Check sheet for the modelled part. Datum: model origin and axes. Units: mm. A direction names the side the tool comes from. Round coordinates to 2 decimals unless told otherwise and drop trailing zeros. Write each loop counter-clockwise with the first axis right and the second up, starting at its lowest first coordinate (ties: lowest second). Pieces come first, ordered by that corner, then holes. Notation, with made-up numbers: (-11.5, 64) -> (47.5, 64) arc R29 ccw to (47.5, 96) -> close; hole circle Ø4 at (40.5, 77.25). An arc over 180 degrees is marked (long way). Answer as a JSON object with one key per item and string values. Group by question number.
```python
from build123d import *

# Parameters (mm, degrees)
CROQUIS2_W              = 85
CROQUIS2_H              = 85
SALIENTE_EXTRUIR1_DEPTH = 110
CROQUIS3_W              = 20
CROQUIS3_H              = 85
CROQUIS3_W_2            = 7
CORTAR_EXTRUIR1_DEPTH   = 2
CROQUIS5_W              = 83
CROQUIS5_H              = 20
CROQUIS5_H_2            = 7
CORTAR_EXTRUIR2_DEPTH   = 2
CROQUIS6_W              = 20
CROQUIS6_H              = 83
CROQUIS6_W_2            = 7
CORTAR_EXTRUIR3_DEPTH   = 2
CROQUIS7_W              = 81
CROQUIS7_H              = 20
CROQUIS7_H_2            = 7
CORTAR_EXTRUIR4_DEPTH   = 2
CORTAR_EXTRUIR6_DEPTH   = 2
CROQUIS12_W             = 9
CROQUIS12_H             = 9
CORTAR_EXTRUIR7_DEPTH   = 2.5
SALIENTE_EXTRUIR3_DEPTH = 10
SALIENTE_EXTRUIR4_DEPTH = 10
SALIENTE_EXTRUIR5_DEPTH = 10
CROQUIS20_W             = 10
CROQUIS20_H             = 10
SALIENTE_EXTRUIR6_DEPTH = 25
CROQUIS21_W             = 150.699966202
CROQUIS21_H             = 120.747177889
CORTAR_EXTRUIR9_DEPTH   = 112
CROQUIS22_W             = 210
CROQUIS22_H             = 195
SALIENTE_EXTRUIR7_DEPTH = 15
CROQUIS23_W             = 208
CROQUIS23_H             = 195
CROQUIS23_W_2           = 188
CROQUIS23_H_2           = 175
EXTRUIR_L_MINA1_DEPTH   = 110
SALIENTE_EXTRUIR8_REACH = 234.166
CROQUIS25_R             = 15
SALIENTE_EXTRUIR8_DRAFT = -10
CROQUIS26_R             = 5
SALIENTE_EXTRUIR9_DEPTH = 10


with BuildPart() as part:
    # Croquis2 → Saliente-Extruir1 (new body)
    with BuildSketch(Plane.XY):
        Rectangle(CROQUIS2_W, CROQUIS2_H)
    extrude(amount=SALIENTE_EXTRUIR1_DEPTH)

    # Croquis3 → Cortar-Extruir1 (cut)
    with BuildSketch(Plane.ZY.offset(42.5)):
        with Locations((100, 0)):
            Rectangle(CROQUIS3_W, CROQUIS3_H)
        with Locations((81.5, 0)):
            Rectangle(CROQUIS3_W_2, CROQUIS3_H)
        with Locations((69.5, 0)):
            Rectangle(CROQUIS3_W_2, CROQUIS3_H)
    extrude(amount=-CORTAR_EXTRUIR1_DEPTH, mode=Mode.SUBTRACT)

    # Croquis5 → Cortar-Extruir2 (cut)
    with BuildSketch(Plane(origin=(0, 42.5, 0), x_dir=(1, 0, 0), z_dir=(0, 1, 0))):
        with Locations((1, -100)):
            Rectangle(CROQUIS5_W, CROQUIS5_H)
        with Locations((1, -81.5)):
            Rectangle(CROQUIS5_W, CROQUIS5_H_2)
        with Locations((1, -69.5)):
            Rectangle(CROQUIS5_W, CROQUIS5_H_2)
    extrude(amount=-CORTAR_EXTRUIR2_DEPTH, mode=Mode.SUBTRACT)

    # Croquis6 → Cortar-Extruir3 (cut)
    with BuildSketch(Plane(origin=(42.5, 0, 0), x_dir=(0, 0, -1), z_dir=(1, 0, 0))):
        with Locations((-100, -1)):
            Rectangle(CROQUIS6_W, CROQUIS6_H)
        with Locations((-81.5, -1)):
            Rectangle(CROQUIS6_W_2, CROQUIS6_H)
        with Locations((-69.5, -1)):
            Rectangle(CROQUIS6_W_2, CROQUIS6_H)
    extrude(amount=-CORTAR_EXTRUIR3_DEPTH, mode=Mode.SUBTRACT)

    # Croquis7 → Cortar-Extruir4 (cut)
    with BuildSketch(Plane(origin=(0, -42.5, 0), x_dir=(-1, 0, 0), z_dir=(0, -1, 0))):
        with Locations((0, -100)):
            Rectangle(CROQUIS7_W, CROQUIS7_H)
        with Locations((0, -81.5)):
            Rectangle(CROQUIS7_W, CROQUIS7_H_2)
        with Locations((0, -69.5)):
            Rectangle(CROQUIS7_W, CROQUIS7_H_2)
    extrude(amount=-CORTAR_EXTRUIR4_DEPTH, mode=Mode.SUBTRACT)

    # Croquis8 → Cortar-Extruir6 (cut)
    with BuildSketch(Plane(origin=(0, 0, 0), x_dir=(-1, 0, 0), z_dir=(0, 0, -1))):
        Polygon((-19.5, -22.5), (-19.5, -1.5), (-28.5, -1.5), (-28.5, 7.5), (-42.5, 7.5), (-42.5, -22.5), align=None)
        Polygon((42.5, -22.5), (42.5, 7.5), (28.5, 7.5), (28.5, -1.5), (19.5, -1.5), (19.5, -22.5), align=None)
    extrude(amount=-CORTAR_EXTRUIR6_DEPTH, mode=Mode.SUBTRACT)

    # Croquis12 → Cortar-Extruir7 (cut)
    with BuildSketch(Plane(origin=(0, 0, 0), x_dir=(-1, 0, 0), z_dir=(0, 0, -1))):
        with Locations((-24, 3)):
            Rectangle(CROQUIS12_W, CROQUIS12_H)
        with Locations((24, 3)):
            Rectangle(CROQUIS12_W, CROQUIS12_H)
    extrude(amount=-CORTAR_EXTRUIR7_DEPTH, mode=Mode.SUBTRACT)

    # Croquis15 → Saliente-Extruir3 (add)
    with BuildSketch(Plane(origin=(-11, 0, 0), x_dir=(0, 0, -1), z_dir=(1, 0, 0))):
        Polygon((0, 17), (18.5, 17), (18.5, 25.5), (28.5, 25.5), (28.5, 34), (10, 34), (10, 25.5), (0, 25.5), align=None)
    extrude(amount=-SALIENTE_EXTRUIR3_DEPTH)

    # Croquis18 → Saliente-Extruir4 (add)
    with BuildSketch(Plane(origin=(11, 0, 0), x_dir=(0, 0, -1), z_dir=(1, 0, 0))):
        Polygon((18.5, 17), (18.5, 25.5), (28.5, 25.5), (28.5, 34), (10, 34), (10, 25.5), (0, 25.5), (0, 17), align=None)
    extrude(amount=SALIENTE_EXTRUIR4_DEPTH)

    # Croquis19 → Saliente-Extruir5 (add)
    with BuildSketch(Plane(origin=(0, 42.5, 0), x_dir=(1, 0, 0), z_dir=(0, 1, 0))):
        Polygon((60.5, -59.370690979), (49.5, -59.370690979), (49.5, -52.370690979), (42.5, -52.370690979), (42.5, -24.05242538), (49.5, -24.05242538), (49.5, -17.05242538), (60.5, -17.05242538), (60.5, -24.05242538), (71.5, -24.05242538), (71.5, -31.05242538), (82.5, -31.05242538), (82.5, -38.05242538), (89.5, -38.05242538), (89.5, -58.05242538), (82.5, -58.05242538), (82.5, -73.370690979), (71.5, -73.370690979), (71.5, -66.370690979), (60.5, -66.370690979), align=None)
        Polygon((-49.5, -17.05242538), (-60.5, -17.05242538), (-60.5, -24.05242538), (-71.5, -24.05242538), (-71.5, -31.05242538), (-82.5, -31.05242538), (-82.5, -38.05242538), (-89.5, -38.05242538), (-89.5, -58.05242538), (-82.5, -58.05242538), (-82.5, -73.370690979), (-71.5, -73.370690979), (-71.5, -66.370690979), (-60.5, -66.370690979), (-60.5, -59.370690979), (-49.5, -59.370690979), (-49.5, -52.370690979), (-42.5, -52.370690979), (-42.5, -24.05242538), (-49.5, -24.05242538), align=None)
    extrude(amount=-SALIENTE_EXTRUIR5_DEPTH)

    # Croquis20 → Saliente-Extruir6 (add)
    with BuildSketch(Plane(origin=(0, -42.5, 0), x_dir=(-1, 0, 0), z_dir=(0, -1, 0))):
        with Locations((-29.5, -25)):
            Rectangle(CROQUIS20_W, CROQUIS20_H)
        with Locations((29.5, -25)):
            Rectangle(CROQUIS20_W, CROQUIS20_H)
        with Locations((-29.5, -60)):
            Rectangle(CROQUIS20_W, CROQUIS20_H)
        with Locations((29.5, -60)):
            Rectangle(CROQUIS20_W, CROQUIS20_H)
    extrude(amount=SALIENTE_EXTRUIR6_DEPTH)

    # Croquis21 → Cortar-Extruir9 (cut)
    with BuildSketch(Plane(origin=(0, 0, 0), x_dir=(0, 0, -1), z_dir=(1, 0, 0))):
        with Locations((-39.284674443, -15.603112065)):
            Rectangle(CROQUIS21_W, CROQUIS21_H)
    extrude(amount=CORTAR_EXTRUIR9_DEPTH, mode=Mode.SUBTRACT)

    # Croquis22 → Saliente-Extruir7 (add)
    with BuildSketch(Plane(origin=(0, 0, 0), x_dir=(0, 0, -1), z_dir=(1, 0, 0))):
        with Locations((-44, 0)):
            Rectangle(CROQUIS22_W, CROQUIS22_H)
    extrude(amount=SALIENTE_EXTRUIR7_DEPTH)

    # Croquis23 → Extruir-Lámina1 (add)
    with BuildSketch(Plane.ZY):
        with Locations((44, 0)):
            Rectangle(CROQUIS23_W, CROQUIS23_H)
        with Locations((44, 0)):
            Rectangle(CROQUIS23_W_2, CROQUIS23_H_2, mode=Mode.SUBTRACT)
    extrude(amount=EXTRUIR_L_MINA1_DEPTH)




with BuildPart() as saliente_extruir8_long_prism_1:
    # Croquis25 → Saliente-Extruir8 (the long prism of profile 1, to be tilted and cut off)
    with BuildSketch(Plane(origin=(0, 42.5, 0), x_dir=(1, 0, 0), z_dir=(0, 1, 0))):
        with Locations((0, -37)):
            Circle(CROQUIS25_R)
    extrude(amount=SALIENTE_EXTRUIR8_REACH)
    saliente_extruir8_tool1_sides = [saliente_extruir8_long_prism_1.faces().sort_by_distance(p)[0] for p in [
        (-15, 159.583, 37),
    ]]
    draft(saliente_extruir8_tool1_sides, Plane(origin=(0, 42.5, 0), x_dir=(1, 0, 0), z_dir=(0, 1, 0)), SALIENTE_EXTRUIR8_DRAFT)  # the draft: side faces tilted about the start plane


with BuildPart() as part_1:
    add(part.part)
    saliente_extruir8_tool1 = saliente_extruir8_long_prism_1.part - part.part
    add(saliente_extruir8_tool1.solids().sort_by_distance((0, 42.5, 37))[0])

    # Barrer2: sweep along a path in Croquis35
    with BuildLine(Plane(origin=(0, 0, 0), x_dir=(0, 0, -1), z_dir=(1, 0, 0))) as barrer2_path:
        Line((-6, 42.5), (10, 87.5))
    # Croquis26 → Barrer2 (sweep)
    with BuildSketch(Plane(origin=(0, 42.5, 0), x_dir=(1, 0, 0), z_dir=(0, 1, 0))):
        with Locations((0, -6)):
            Circle(CROQUIS26_R)
    sweep(path=barrer2_path.line)

    # Croquis37 → Saliente-Extruir9 (add)
    with BuildSketch(Plane.ZY):
        with BuildLine():
            Line((105, -53.5), (117, -53.5))
            Line((117, -53.5), (117, 55.5))
            Line((117, 55.5), (105, 55.5))
            ThreePointArc((105, 55.5), (97, 63.5), (105, 71.5))
            Line((105, 71.5), (125, 71.5))
            ThreePointArc((125, 71.5), (130.656854249, 69.156854249), (133, 63.5))
            Line((133, 63.5), (133, -61.5))
            ThreePointArc((133, -61.5), (130.656854249, -67.156854249), (125, -69.5))
            Line((125, -69.5), (105, -69.5))
            ThreePointArc((105, -69.5), (97, -61.5), (105, -53.5))
        make_face()
        with BuildLine():
            ThreePointArc((-47, 63.5), (-44.656854249, 69.156854249), (-39, 71.5))
            Line((-39, 71.5), (-19, 71.5))
            ThreePointArc((-19, 71.5), (-11, 63.5), (-19, 55.5))
            Line((-19, 55.5), (-31, 55.5))
            Line((-31, 55.5), (-31, -53.5))
            Line((-31, -53.5), (-19, -53.5))
            ThreePointArc((-19, -53.5), (-11, -61.5), (-19, -69.5))
            Line((-19, -69.5), (-39, -69.5))
            ThreePointArc((-39, -69.5), (-44.656854249, -67.156854249), (-47, -61.5))
            Line((-47, -61.5), (-47, 63.5))
        make_face()
    extrude(amount=SALIENTE_EXTRUIR9_DEPTH)


solid = part_1.part
```
(1) Release check for a two-part mould opening along Y. For faces 1 (the flat face through (-48, -97.5, 45)), 2 (the flat face through (-42, 0, 90)), 3 (the flat face through (-48, 97.5, 45)) record: pulls with the +Y half, pulls with the -Y half, needs draft (parallel to the pull), parting line crosses it, or undercut.
(2) Scan lines: line 1 along Z through (x, y) = (-18, 8); line 2 along Y through (x, z) = (-62, 56); line 3 along Y through (x, z) = (-34, 58). Record each from-to range of solid material in increasing order.
(3) Section check A-A on x = -56. Record the cut outline in (y, z), then the cut area to 3 significant figures.
(4) Access from +Z, -Z, +X, -X, +Y, -Y to the whole of each face (thin tool, end or side, straight path). Record for faces 4 (the flat face through (0, 65, 9)), 5 (the flat face through (-54, -1, 148)).
(5) Go/stop test with flat-tipped pins: pin 1 Ø6 at (y, z) = (-34.5, -2.5) entering from -X; pin 2 Ø12 at (y, z) = (60.5, -9) entering from -X; pin 3 Ø6 at (x, y) = (-22.5, -67) entering from -Z. Record where each tip stops, or that it passes through.
Data:
{
 "1": {"face 1": "pulls with the -Y half", "face 2": "undercut", "face 3": "pulls with the +Y half"},
 "2": {"line 1": "z = -60 to -50, 0 to 110, 138 to 148", "line 2": "y = -97.5 to -87.5, 32.5 to 42.5, 87.5 to 97.5", "line 3": "y = -97.5 to -87.5, -67.5 to 42.5, 87.5 to 97.5"},
 "3": {"outline": "(-97.5, -60) -> (97.5, -60) -> (97.5, 148) -> (-97.5, 148) -> close; (32.5, 17.05) -> (42.5, 17.05) -> (42.5, 59.37) -> (32.5, 59.37) -> close; hole (-87.5, -50) -> (87.5, -50) -> (87.5, 138) -> (-87.5, 138) -> close", "area": "8,080 mm²"},
 "4": {"face 4": "-X", "face 5": "+Z, -X, +Y, -Y"},
 "5": {"pin 1": "stops at x = -42.5", "pin 2": "stops at x = -10", "pin 3": "stops at z = -60"}
}
